Can you work these out from the model? Positions are in its coordinate system, mm. A direction names the side the tool comes from. Round coordinates to 2 decimals unless told otherwise and drop trailing zeros. Loops run counter-clockwise (first coordinate to the right, second up) from the corner with the lowest first, then second, coordinate; pieces in that order, holes last. Notation, with made-up numbers: (-5.75, 55) -> (32.25, 55) arc R23 cw to (32.25, 68) -> close; hole circle Ø1 at (71, 76.5). An arc over 180 degrees is marked (long way). Use a Markdown table: item, result.
from build123d import *

# Parameters (mm, degrees)
SKETCH1_R   = 1.5
BOARD_DEPTH = 1.5


with BuildPart() as part:
    # Sketch1 → board (new body)
    with BuildSketch(Plane(origin=(0, 0, 0), x_dir=(1, 0, 0), z_dir=(0, 1, 0))):
        with BuildLine():
            Line((0, 34.5), (-26, 34.5))
            Line((-26, 34.5), (-26, 31.5))
            ThreePointArc((-26, 31.5), (-30, 27.5), (-34, 31.5))
            Line((-34, 31.5), (-34, 34.5))
            Line((-34, 34.5), (-57.5, 34.5))
            ThreePointArc((-57.5, 34.5), (-80.43741485, 25.77062281), (-91.767331381, 4))
            Line((-91.767331381, 4), (-89, 4))
            ThreePointArc((-89, 4), (-85, 0), (-89, -4))
            Line((-89, -4), (-91.767331381, -4))
            ThreePointArc((-91.767331381, -4), (-80.43741485, -25.77062281), (-57.5, -34.5))
            Line((-57.5, -34.5), (-41.5, -34.5))
            ThreePointArc((-41.5, -34.5), (-38.424621202, -27.075378798), (-31, -24))
            Line((-31, -24), (-31, -11.5))
            Line((-31, -11.5), (31, -11.5))
            Line((31, -11.5), (31, -24))
            ThreePointArc((31, -24), (38.424621202, -27.075378798), (41.5, -34.5))
            Line((41.5, -34.5), (57.5, -34.5))
            ThreePointArc((57.5, -34.5), (80.43741485, -25.77062281), (91.767331381, -4))
            Line((91.767331381, -4), (89, -4))
            ThreePointArc((89, -4), (85, 0), (89, 4))
            Line((89, 4), (91.767331381, 4))
            ThreePointArc((91.767331381, 4), (80.43741485, 25.77062281), (57.5, 34.5))
            Line((57.5, 34.5), (34, 34.5))
            Line((34, 34.5), (34, 31.5))
            ThreePointArc((34, 31.5), (30, 27.5), (26, 31.5))
            Line((26, 31.5), (26, 34.5))
            Line((26, 34.5), (0, 34.5))
        make_face()
        with Locations(Location((-57.5, 0, 0), (0, 0, 270))):
            Circle(SKETCH1_R, mode=Mode.SUBTRACT)
        with Locations(Location((57.5, 0, 0), (0, 0, 270))):
            Circle(SKETCH1_R, mode=Mode.SUBTRACT)
    extrude(amount=BOARD_DEPTH)


solid = part.part
1. I want a section at B-B (y = 0.7). Please give me the cut outline in (x, z).
Answer sheet:
| item | result |
|---|---|
| outline | (-91.77, -4) arc R34.5 ccw to (-57.5, -34.5) -> (-34, -34.5) -> (-34, -31.5) arc R4 cw to (-26, -31.5) -> (-26, -34.5) -> (26, -34.5) -> (26, -31.5) arc R4 cw to (34, -31.5) -> (34, -34.5) -> (57.5, -34.5) arc R34.5 ccw to (91.77, -4) -> (89, -4) arc R4 cw to (89, 4) -> (91.77, 4) arc R34.5 ccw to (57.5, 34.5) -> (41.5, 34.5) arc R10.5 cw to (31, 24) -> (31, 11.5) -> (-31, 11.5) -> (-31, 24) arc R10.5 cw to (-41.5, 34.5) -> (-57.5, 34.5) arc R34.5 ccw to (-91.77, 4) -> (-89, 4) arc R4 cw to (-89, -4) -> close; hole circle Ø3 at (-57.5, 0); hole circle Ø3 at (57.5, 0) |
2. I want a section at A-A (z = 16.5). Please give me the cut outline in (x, y).
Answer sheet:
| item | result |
|---|---|
| outline | (-87.8, 0) -> (-31, 0) -> (-31, 1.5) -> (-87.8, 1.5) -> close; (31, 0) -> (87.8, 0) -> (87.8, 1.5) -> (31, 1.5) -> close |
3. Will these pins go through, and if not, where does the flat tip stop? pin 1 Ø0.8 at (x, y) = (-11, 1) entering from +Z; pin 2 Ø1.8 at (x, z) = (57.5, 0) entering from +Y.
Answer sheet:
| item | result |
|---|---|
| pin 1 | stops at z = 11.5 |
| pin 2 | passes through |
4. Which directions (+Z, -Z, +X, -X, +Y, -Y) give clear straight access to the entire face, cutting with the end or side of a thin tool? Please do faces 1 (the cylindrical face through (-56, 1, 0)), 2 (the cylindrical face through (-38.51, 0.74, 27.16)).
Answer sheet:
| item | result |
|---|---|
| face 1 | +Y, -Y |
| face 2 | +Z, +Y, -Y |
5. If we mould it in two halves opening along Z, with no side actions, what happens to faces 3 (the cylindrical face through (38.34, 0.74, 26.99)), 4 (the cylindrical face through (59, 1, 0)), 5 (the cylindrical face through (-80.174, 0.74, -26.003)), 6 (the cylindrical face through (85, 1, 0))? For each: +Z half, -Z half, draft (parallel to the pull), parting line (faces both ways), or undercut.
Answer sheet:
| item | result |
|---|---|
| face 3 | +Z half |
| face 4 | undercut |
| face 5 | -Z half |
| face 6 | undercut |
6. I want a section at C-C (x = 12.5). Please give me the cut outline in (y, z), plus the area to 3 significant figures.
Answer sheet:
| item | result |
|---|---|
| outline | (0, -34.5) -> (1.5, -34.5) -> (1.5, 11.5) -> (0, 11.5) -> close |
| area | 69.0 mm² |
7. I want a section at D-D (z = -25). Please give me the cut outline in (x, y), plus the area to 3 significant figures.
Answer sheet:
| item | result |
|---|---|
| outline | (-81.27, 0) -> (81.27, 0) -> (81.27, 1.5) -> (-81.27, 1.5) -> close |
| area | 244 mm² |
8. I need wall thicknesses on line 1 (X direction, y = 1.25, z = 0); line 2 (X direction, y = 0.15, z = 25.5); line 3 (X direction, y = 0.9, z = 15). Which ranges of each line are inside material? Lowest first, please.
Answer sheet:
| item | result |
|---|---|
| line 1 | x = -85 to -59, -56 to 56, 59 to 85 |
| line 2 | x = -80.74 to -36.41, 36.41 to 80.74 |
| line 3 | x = -88.57 to -31, 31 to 88.57 |
